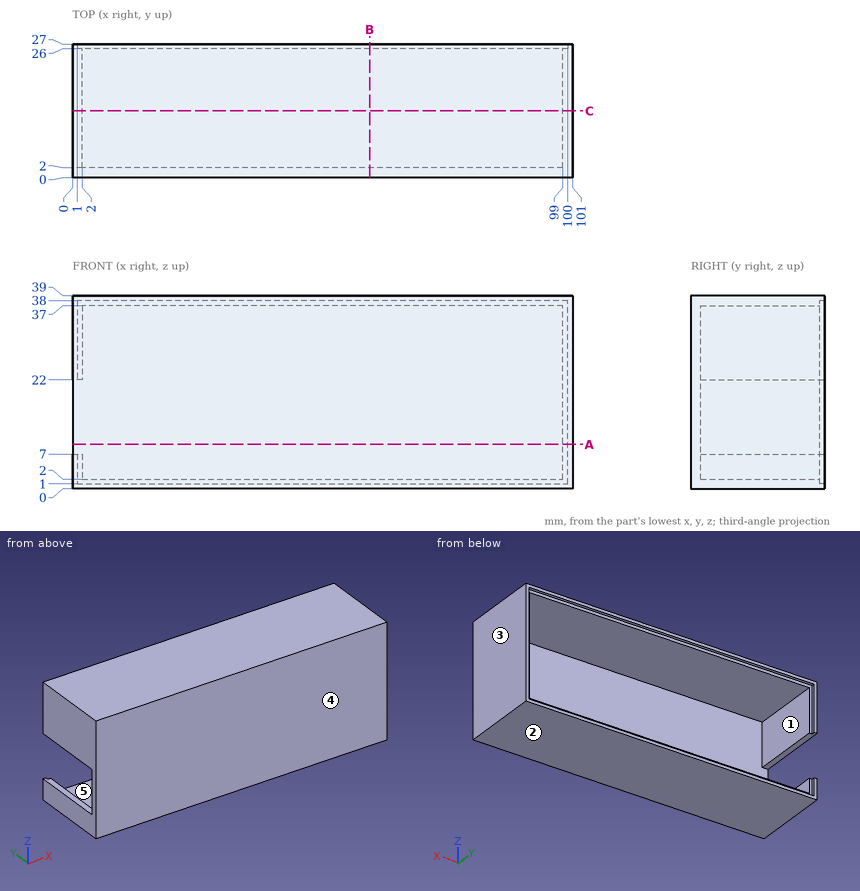
Study the drawing (mm; zero at the part's minimum x, y, z) and answer. A direction names the side the tool comes from. Give positions to 0.01 mm unless a question says otherwise; leave off trailing zeros. Loops run counter-clockwise (first coordinate to the right, second up) from the corner with the lowest first, then second, coordinate; pieces in that order, holes last. Notation, with made-up numbers: (76, 11) - (114, 11) arc R18 cw to (114, 33) - close; hole circle Ø3 at (6, 75.25). An arc over 180 degrees is marked (long way). Answer in a Markdown table with one row per item. Add a question column.
Q1. A tool of negligible diameter and unlimited length cuts with its end or side. For the marked faces 4 and 5, from which of +Z, -Z, +X, -X, +Y, -Y can it reach the whole face along a straight path? Write none if from no direction.
Q2. The part is cut by section B-B (x = 60). Determine the outline of the cut face in (y, z), and give its area (3 significant figures).
Q3. Consider line 1 along X through (y, z) = (8.5, 4.5); line 2 along Z through (x, y) = (61.5, 2.5); line 3 along Y through (x, z) = (93.5, 5). Determine where each line is inside the solid, lowest interval first.
Q4. Each of these flat-tipped pins is pushed along its axis until it touches: P1, Ø2, axis at x = 83, z = 6, coming from the +Y side; P2, Ø0.5, axis at y = 26.5, z = 13, coming from the -X side; P3, Ø7, axis at y = 17.5, z = 18, coming from the -X side. Where does it stop, or does it pass through?
Q5. Determine the mould class of the marked faces 1, 2 and 3 for opening direction X: released by +X, released by -X, zero draft, split by the parting line, or undercut.
Q6. The part is cut by section A-A (z = 9). Determine the outline of the cut face in (x, y), and give its area (3 significant figures).
Q7. The part is cut by section C-C (y = 13.5). Determine the outline of the cut face in (x, z).
Solution:
| question | item | result |
|---|---|---|
| 1 | face 4 | +Z, -Z, +X, -X, -Y |
| 1 | face 5 | +Y |
| 2 | outline | (0, 0) - (27, 0) - (27, 1) - (26, 1) - (26, 2) - (2, 2) - (2, 37) - (26, 37) - (26, 38) - (27, 38) - (27, 39) - (0, 39) - close |
| 2 | area | 176 mm² |
| 3 | line 1 | x = 0 to 2, 99 to 101 |
| 3 | line 2 | z = 0 to 2, 37 to 39 |
| 3 | line 3 | y = 0 to 2 |
| 4 | P1 | stops at y = 2 |
| 4 | P2 | stops at x = 100 |
| 4 | P3 | stops at x = 99 |
| 5 | face 1 | undercut |
| 5 | face 2 | zero draft |
| 5 | face 3 | released by +X |
| 6 | outline | (0, 0) - (101, 0) - (101, 27) - (100, 27) - (100, 26) - (99, 26) - (99, 2) - (0, 2) - close |
| 6 | area | 251 mm² |
| 7 | outline | (0, 0) - (101, 0) - (101, 39) - (0, 39) - (0, 22) - (2, 22) - (2, 37) - (99, 37) - (99, 2) - (2, 2) - (2, 7) - (0, 7) - close |
